from build123d import *

# Parameters (mm, degrees)
F2_R     = 4.7625
F3_DEPTH = 25.4


with BuildPart() as f1:
    # F0 (on Front) → F1 (revolve)
    with BuildSketch(Plane.XZ):
        Polygon((-152.4, 0), (0, 0), (0, 7.112), (-1.5748, 8.6868), (-22.987, 8.6868), (-22.987, 12.7), (-152.4, 12.7), align=None)
    revolve(axis=Axis((-76.2, 0, 0), (1, 0, 0)))

    # F2 (on Top) → F3 (cut)
    with BuildSketch(Plane.XY):
        with Locations((-25.4, 0)):
            Circle(F2_R)
    extrude(amount=F3_DEPTH, mode=Mode.SUBTRACT)


solid = f1.part
CAD build for the part. Positions are in the model's coordinates, mm. A direction names the side the tool comes from. Round coordinates to 2 decimals unless told otherwise and drop trailing zeros. Order: outer loops, then holes, each group sorted by start corner. A loop starts at its lowest first (then second) coordinate and runs counter-clockwise, first axis right, second up. Notation, with made-up numbers: (55.5, 35) - (71.5, 35) arc R12 cw to (71.5, 45) - close; hole circle Ø7 at (2, 12). An arc over 180 degrees is marked (long way). Return JSON: item names as keys, results as strings.
(1) Cut at C-C (y = 11). Give the cut face in (x, z).
Answer key:
{"outline": "(-152.4, -6.35) - (-22.99, -6.35) - (-22.99, 6.35) - (-152.4, 6.35) - close"}
(2) Cut at A-A (y = 0). Give the cut face in (x, z).
Answer key:
{"outline": "(-152.4, -12.7) - (-22.99, -12.7) - (-22.99, -8.69) - (-1.57, -8.69) - (0, -7.11) - (0, 7.11) - (-1.57, 8.69) - (-20.64, 8.69) - (-20.64, 0) - (-30.16, 0) - (-30.16, 12.7) - (-152.4, 12.7) - close"}
(3) Cut at D-D (x = -25.4). Give the cut face in (y, z).
Answer key:
{"outline": "(-4.76, 0) - (-4.76, 11.77) arc R12.7 ccw (long way) to (4.76, 11.77) - (4.76, 0) - close"}
(4) Cut at B-B (x = -136). Give the cut face in (y, z), then the cut area to 3 significant figures.
Answer key:
{"outline": "circle Ø25.4 at (0, 0)", "area": "507 mm^2"}
(5) Tool access for faces 5 (the face through (-88.6, 12.4, -2.75)), 6 (the face through (-22.987, -3, -8.4)): list every direction of +Z, -Z, +X, -X, +Y, -Y with a clear straight run to the whole face (end or side of a thin tool).
Answer key:
{"face 5": "+X, -X", "face 6": "+X"}
(6) Pin check, flat tips, straight feed: pin 1 Ø12 at (x, y) = (-45.5, 9) entering from +Z; pin 2 Ø5 at (x, z) = (-32.5, -8.5) entering from +Y; pin 3 Ø3 at (x, y) = (-27, 1) entering from +Z. Stop position of each tip, or through.
Answer key:
{"pin 1": "stops at z = 12.34", "pin 2": "stops at y = 11.19", "pin 3": "stops at z = 0"}
(7) Pull direction Y, two halves, no side cores. Call faces 1 (the face through (-12.43, -0.38, -8.68)), 2 (the face through (0, 0, 0)), 3 (the face through (-25, 0, 0)), 4 (the face through (-29.18, -2.9, 4.85)): +Y half, -Y half, draft (parallel to the pull), parting line (faces both ways), or undercut.
Answer key:
{"face 1": "parting line", "face 2": "draft", "face 3": "undercut", "face 4": "undercut"}
(8) Wall check: probe 1 along X at (y, z) = (0, 7); probe 2 along X at (y, z) = (0, 10.25); probe 3 along X at (y, z) = (-7.75, -8.75). Give the ranges that are in metal, low to high. Write a range as from..to.
Answer key:
{"probe 1": "x = -152.4..-30.16, -20.64..0", "probe 2": "x = -152.4..-30.16", "probe 3": "x = -152.4..-22.99"}
